Input: part model. Units: mm. Frame: model coordinates. Coordinates: 2 decimals unless noted, no trailing zeros. Write each loop counter-clockwise with the first axis right and the second up, starting at its lowest first coordinate (ties: lowest second). Pieces come first, ordered by that corner, then holes. Notation, with made-up numbers: M 48,-33 L 65,-33 A12 cw 65,-18 Z; hole C 80,73 d5. An arc over 180 degrees is marked long. Use one line per item in the form item = value.
from build123d import *

# Parameters (mm, degrees)
EXTRUDE1_DEPTH = 3.175
EXTRUDE2_DEPTH = 3.175
SKETCH4_R      = 4.750719405
EXTRUDE3_DEPTH = 184.514359856


with BuildPart() as part:
    # Sketch1 → Extrude1 (new body)
    with BuildSketch(Plane(origin=(0, 0, 0), x_dir=(1, 0, 0), z_dir=(0, 1, 0))):
        with BuildLine():
            Line((0, 0), (152.4, 0))
            Line((152.4, 0), (152.4, 95.25))
            ThreePointArc((152.4, 95.25), (150.540128061, 99.740128061), (146.05, 101.6))
            Line((146.05, 101.6), (6.35, 101.6))
            ThreePointArc((6.35, 101.6), (1.859871939, 99.740128061), (0, 95.25))
            Line((0, 95.25), (0, 0))
        make_face()
    extrude(amount=-EXTRUDE1_DEPTH)

    # Sketch2 → Extrude2 (add)
    with BuildSketch(Plane(origin=(0, 0, 0), x_dir=(1, 0, 0), z_dir=(0, 1, 0))):
        Polygon((43.041816565, 25.4), (37.395908282, 35.179), (26.104091718, 35.179), (20.458183435, 25.4), (26.104091718, 15.621), (37.395908282, 15.621), align=None)
    extrude(amount=EXTRUDE2_DEPTH)

    # Sketch3 → Revolve1 (revolve)
    with BuildSketch(Plane.XY.offset(-25.4), mode=Mode.PRIVATE) as revolve1_sk:
        with BuildLine():
            Line((31.75, 8.191629817), (37.811630026, 8.191629817))
            ThreePointArc((37.811630026, 8.191629817), (39.423025401, 5.879728861), (40.214178276, 3.175))
            Line((40.214178276, 3.175), (31.75, 3.175))
            Line((31.75, 3.175), (31.75, 8.191629817))
        make_face()
    revolve(revolve1_sk.sketch.rotate(Axis((31.75, 3.175, -25.4), (0, 1, 0)), 270), axis=Axis((31.75, 3.175, -25.4), (0, 1, 0)))

    # Sketch4 → Extrude3 (cut, through all)
    with BuildSketch(Plane(origin=(0, 8.191629817, 0), x_dir=(-1, 0, 0), z_dir=(0, 1, 0))):
        with Locations(Location((-31.75, -25.4, 0), (0, 0, 90))):
            Circle(SKETCH4_R)
    extrude(amount=-EXTRUDE3_DEPTH, mode=Mode.SUBTRACT)


solid = part.part
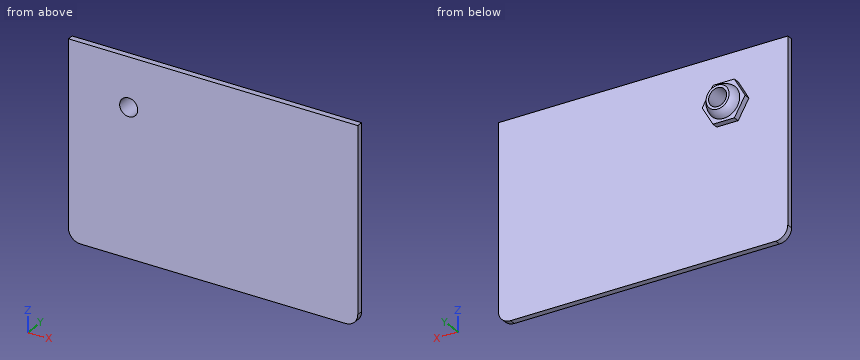
(1) First-contact query: pin 1 Ø2.5 at (x, y) = (29.5, 1.5) entering from +Z. Flat tip, straight axial feed; report the tip coordinate or a pass-through.
Computed:
pin_1 = -15.62
(2) Section query B-B on x = 75. Return the cut outline in (y, z) (3 decimals), plus the area to 3 significant figures.
Computed:
outline = M -3.175,-101.6 L 0,-101.6 L 0,0 L -3.175,0 Z
area = 323 mm^2
(3) Section query A-A on z = -67.5. Return the cut outline in (x, y) (3 decimals).
Computed:
outline = M 0,-3.175 L 152.4,-3.175 L 152.4,0 L 0,0 Z
(4) Line query: probe 1 along Y at (x, z) = (138.5, -53.5) (3 decimals); probe 2 along X at (y, z) = (4.25, -25.4); probe 3 along X at (y, z) = (4, -25.4). Output: solid intervals per line, ascending.
Computed:
probe_1 = -3.175 to 0
probe_2 = 23.49 to 27, 36.5 to 40.01
probe_3 = 23.43 to 27, 36.5 to 40.07
